Autodesk Inventor part; units mm, degrees
ref_plane "YZ Plane" through (0, 0, 0) normal (1, 0, 0) x (0, 1, 0)
ref_plane "XZ Plane" through (0, 0, 0) normal (0, 1, 0) x (-1, 0, 0)
ref_plane "XY Plane" through (0, 0, 0) normal (0, 0, 1) x (1, 0, 0)
sketch "スケッチ1" plane through (0, 0, 0) normal (0, 1, 0) x (-1, 0, 0)
  line L0 (25, 0) -> (-25, 0)
  line L1 (-25, 0) -> (-25, -104.5)
  line L2 (-25, -104.5) -> (25, -104.5) construction
  line L3 (25, -104.5) -> (25, 0)
  circle A0 centre (0, 0) radius 25
  circle A1 centre (0, 0) radius 57 construction
  circle A2 centre (0, -79.5) radius 22.5 construction
  circle A3 centre (0, 0) radius 75 construction
  circle A4 centre (0, -79.5) radius 10.75
  circle A5 centre (0, 0) radius 10.75
  circle A6 centre (-77.7461, -62.8931) radius 25
  circle A7 centre (-77.7461, -62.8931) radius 10.75
  circle A8 centre (0, -79.5) radius 25
  line L4 (-5.2223, -103.9485) -> (-82.9684, -87.3415)
  line L5 (-72.5238, -38.4446) -> (5.2223, -55.0515)
  line L6 (-77.7461, -62.8931) -> (-82.9684, -87.3415)
  point P0 (25, -79.5)
  point P1 (-25, -48.5959)
  dimension "d0" = 114
  dimension "d1" = 45
  dimension "d2" = 150
  dimension "d4" = 21.5
  dimension "d5" = 50
  dimension "d25" = 79.5
extrude "押し出し1" add sketch "スケッチ1" along normal blind 5.5 contours A0 L0 A5 | L0 A5 A0 | L3 A8 L5 L1 A0 | A8 | A8 L1 L5 | L4 L1 A8 | L1 L4 A6 L5 | A6
sketch "スケッチ4" plane through (0, 5.5, 0) normal (0, 1, 0) x (1, 0, 0)
  line L0 (-1, 90.2034) -> (1, 90.2034)
  line L1 (1, 90.2034) -> (1, 96.5)
  line L2 (1, 96.5) -> (-1, 96.5)
  line L3 (-1, 96.5) -> (-1, 90.2034)
  arc A0 (-25, 0) -> (25, 0) centre (0, 0) ccw
  line L4 (25, 0) -> (25, 48.5959)
  line L5 (25, 48.5959) -> (72.5238, 38.4446)
  arc A1 (72.5238, 38.4446) -> (82.9684, 87.3415) centre (77.7461, 62.8931) ccw
  line L6 (82.9684, 87.3415) -> (5.2223, 103.9485)
  arc A2 (5.2223, 103.9485) -> (-25, 79.5) centre (0, 79.5) ccw
  line L7 (-25, 79.5) -> (-25, 0)
  circle A3 centre (0, 0) radius 10.75
  circle A4 centre (77.7461, 62.8931) radius 10.75
  circle A5 centre (0, 79.5) radius 10.75
  circle A6 centre (0, 79.5) radius 10.75
  line L8 (-16.9706, -1) -> (16.9706, -1)
  line L9 (16.9706, -1) -> (16.9706, 1)
  line L10 (16.9706, 1) -> (-16.9706, 1)
  line L11 (-16.9706, 1) -> (-16.9706, -1)
  line L12 (-1, -16.9706) -> (1, -16.9706)
  line L13 (1, -16.9706) -> (1, 16.9706)
  line L14 (1, 16.9706) -> (-1, 16.9706)
  line L15 (-1, 16.9706) -> (-1, -16.9706)
  circle A7 centre (0, 0) radius 17
  line L16 (94.7167, 63.8931) -> (60.7756, 63.8931)
  line L17 (60.7756, 63.8931) -> (60.7756, 61.8931)
  line L18 (60.7756, 61.8931) -> (94.7167, 61.8931)
  line L19 (94.7167, 61.8931) -> (94.7167, 63.8931)
  line L20 (78.7461, 79.8636) -> (76.7461, 79.8636)
  line L21 (76.7461, 79.8636) -> (76.7461, 45.9225)
  line L22 (76.7461, 45.9225) -> (78.7461, 45.9225)
  line L23 (78.7461, 45.9225) -> (78.7461, 79.8636)
  line L24 (16.9706, 80.5) -> (-16.9706, 80.5)
  line L25 (-16.9706, 80.5) -> (-16.9706, 78.5)
  line L26 (-16.9706, 78.5) -> (16.9706, 78.5)
  line L27 (16.9706, 78.5) -> (16.9706, 80.5)
  line L28 (16.9706, 80.5) -> (-16.9706, 78.5) construction
  line L29 (-16.9706, 80.5) -> (16.9706, 78.5) construction
  point P0 (0, 96.5)
  point P1 (-16.9706, 0)
  point P2 (0, 16.9706)
  point P3 (-1, -10.7034)
  point P4 (1, -10.7034)
  point P5 (10.7034, 1)
  point P6 (10.7034, -1)
  point P7 (-1, 10.7034)
  point P8 (1, 10.7034)
  point P9 (-10.7034, -1)
  point P10 (-10.7034, 1)
  point P11 (60.7756, 62.8931)
  point P12 (77.7461, 45.9225)
  point P13 (77.7461, 61.8931)
  point P14 (76.7461, 62.8931)
  point P15 (88.4495, 63.8931)
  point P16 (78.7461, 73.5965)
  point P17 (76.7461, 73.5965)
  point P18 (67.0427, 63.8931)
  point P19 (67.0427, 61.8931)
  point P20 (76.7461, 52.1897)
  point P21 (78.7461, 52.1897)
  point P22 (88.4495, 61.8931)
  dimension "d26" = 17
  dimension "d27" = 2
  dimension "d30" = 34
extrude "押し出し4" cut sketch "スケッチ4" against normal through all contours A5 L0 | L3 L2 L1 A5 | L24 A5 L26 | A5 L26 L25 L24 | L24 L27 L26 A5 | A3 L10 L9 L8 | A3 L15 L14 L13 | L13 L12 L15 A3 | A3 L8 L11 L10 | A4 L18 L23 L16 | A4 L16 L19 L18 | L16 L23 A4 | A4 L23 L18 | L23 L16 L21 A4 | A4 L21 L20 L23 | L23 L18 L21 L16 | L23 L22 L21 A4 | A4 L21 L18 L23 | L21 L16 A4 | L21 L18 A4 L16 | A4 L18 L21 | A4 L18 L17 L16
fillet "フィレット1" radius 5 1 edges at (25, 2.75, -48.5959)
properties part number "gear_plate_1" material "木材 (カエデ材)"
The listing builds one solid part. Answer for the finished solid, in the listing's coordinates (mm). A direction names the side the tool comes from. Round coordinates to 2 decimals unless told otherwise and drop trailing zeros. Loops run counter-clockwise (first coordinate to the right, second up) from the corner with the lowest first, then second, coordinate; pieces in that order, holes last.
Q1. Section A-A, the plane z = 9 is taken. Determine the outline of the cut face in (x, y), then the cut area to 3 significant figures.
Q2. Section B-B, the plane x = -12.5 is taken. Determine the outline of the cut face in (y, z).
Q3. Section D-D, the plane x = 81.5 is taken. Determine the outline of the cut face in (y, z), then the cut area to 3 significant figures.
Q4. For a pull along Z with two mould halves and no side action, classify faces 3 (the face through (25, 3, -21)), 4 (the face through (64, 3, -61.893)), 5 (the face through (-15.964, 2.712, -98.739)) as released by +Z, released by -Z, zero draft, split by the parting line, or undercut.
Q5. Given pin 1 Ø4 at (x, z) = (86, -87.5) entering from -Y; pin 2 Ø3 at (y, z) = (2, 3.5) entering from -X; pin 3 Ø3 at (x, y) = (62.5, 3) entering from +Z; pin 4 Ø1.6 at (y, z) = (3, 14.5) entering from -X, each flat-ended and moving along its own axis, determine where each tip first touches the part or whether it passes through.
Q6. Section C-C, the plane z = -72 is taken. Determine the outline of the cut face in (x, y), then the cut area to 3 significant figures.
Q7. Which of the six approach directions +Z, -Z, +X, -X, +Y, -Y give full straight-line access (tool end or side, diameter ignored) to faces 1 (the face through (0.55, 2.712, 24.994)), 2 (the face through (1, 3, -93))?
Q8. Find the intervals of material crossed by line 1 (Z direction, x = 0, y = 3.6); line 2 (Z direction, x = -3, y = 5.2); line 3 (X direction, y = 1.3, z = 0), in increasing order.
Completed:
1. outline: (-23.32, 0) - (-5.88, 0) - (-5.88, 5.5) - (-23.32, 5.5) - close; (5.88, 0) - (23.32, 0) - (23.32, 5.5) - (5.88, 5.5) - close
1. area: 192 mm2
2. outline: (0, -101.15) - (5.5, -101.15) - (5.5, -80.5) - (0, -80.5) - close; (0, -78.5) - (5.5, -78.5) - (5.5, -1) - (0, -1) - close; (0, 1) - (5.5, 1) - (5.5, 21.65) - (0, 21.65) - close
3. outline: (0, -87.66) - (5.5, -87.66) - (5.5, -72.97) - (0, -72.97) - close; (0, -52.82) - (5.5, -52.82) - (5.5, -38.18) - (0, -38.18) - close
3. area: 161 mm2
4. face 3: zero draft
4. face 4: undercut
4. face 5: released by -Z
5. pin 1: stops at y = 0
5. pin 2: stops at x = -24.92
5. pin 3: stops at z = -40.27
5. pin 4: stops at x = -20.91
6. outline: (-25, 0) - (-7.7, 0) - (-7.7, 5.5) - (-25, 5.5) - close; (7.7, 0) - (72.03, 0) - (72.03, 5.5) - (7.7, 5.5) - close; (83.46, 0) - (101.03, 0) - (101.03, 5.5) - (83.46, 5.5) - close
6. area: 546 mm2
7. face 1: +Z, +Y, -Y
7. face 2: +Y, -Y
8. line 1: z = -104.5 to -96.5, -68.75 to -16.97, 16.97 to 25
8. line 2: z = -104.32 to -89.82, -69.18 to -10.32, 10.32 to 24.82
8. line 3: x = -25 to -16.97, 16.97 to 25
